Autodesk Fusion 360 part; units mm, degrees
sketch "Sketch1" plane through (0, 0, 0) normal (0, 1, 0) x (1, 0, 0)
  line L0 (0, 0) -> (50, 0)
  line L1 (50, 0) -> (50, -50)
  line L2 (50, -50) -> (0, -50)
  line L3 (0, -50) -> (0, 0)
  dimension "d1" = 50
  dimension "d2" = 50
extrude "Extrude1" add sketch "Sketch1" along normal blind 15
sketch "Sketch2" plane through (0, 15, 0) normal (0, 1, 0) x (-1, 0, 0)
  line L0 (0, 50) -> (-50, 50)
  line L1 (-50, 50) -> (-50, 0)
  line L2 (-50, 0) -> (0, 0)
  line L3 (0, 0) -> (0, 50)
  line L4 (-25, 50) -> (-25, 0) construction
  line L5 (0, 25) -> (-50, 25) construction
  line L6 (-46.6959, 41.7465) -> (-42.6959, 41.7465)
  line L7 (-42.6959, 41.7465) -> (-42.6959, 46.7465)
  line L8 (-42.6959, 46.7465) -> (-46.6959, 46.7465)
  line L9 (-46.6959, 46.7465) -> (-46.6959, 41.7465)
  line L10 (-42.6959, 3.2535) -> (-46.6959, 3.2535)
  line L11 (-46.6959, 3.2535) -> (-46.6959, 8.2535)
  line L12 (-46.6959, 8.2535) -> (-42.6959, 8.2535)
  line L13 (-42.6959, 8.2535) -> (-42.6959, 3.2535)
  line L14 (-3.3041, 41.7465) -> (-7.3041, 41.7465)
  line L15 (-3.3041, 46.7465) -> (-3.3041, 41.7465)
  line L16 (-7.3041, 41.7465) -> (-7.3041, 46.7465)
  line L17 (-7.3041, 46.7465) -> (-3.3041, 46.7465)
  line L18 (-7.3041, 8.2535) -> (-7.3041, 3.2535)
  line L19 (-3.3041, 8.2535) -> (-7.3041, 8.2535)
  line L20 (-3.3041, 3.2535) -> (-3.3041, 8.2535)
  line L21 (-7.3041, 3.2535) -> (-3.3041, 3.2535)
  dimension "d5" = 5
  dimension "d6" = 4
extrude "Extrude2" add sketch "Sketch2" along normal blind 50 contours L6 L7 L8 L9 | L10 L11 L12 L13 | L14 L15 L16 L17 | L18 L19 L20 L21
fillet "Fillet1" radius 5 1 edges at (0, 0, 25)
sketch "Sketch3" plane through (0, 0, 0) normal (0, -1, 0) x (1, 0, 0)
  line L0 (5, 50) -> (5, 0)
  line L1 (5, 0) -> (50, 0)
  line L2 (50, 0) -> (50, 50)
  line L3 (50, 50) -> (5, 50)
  line L4 (50, 0) -> (45, 0)
  line L5 (45, 0) -> (45, 50)
  line L6 (45, 50) -> (50, 50)
  line L7 (50, 50) -> (50, 0)
  dimension "d11" = 5
  dimension "d12" = 50
extrude "Extrude3" add sketch "Sketch3" along normal blind 50 contours L1 L2 L3 L4 L5 L6 L7
The listing builds one solid part. Answer for the finished solid, in the listing's coordinates (mm). A direction names the side the tool comes from. Coordinates: 2 decimals unless noted, no trailing zeros. Write each loop counter-clockwise with the first axis right and the second up, starting at its lowest first coordinate (ties: lowest second). Pieces come first, ordered by that corner, then holes. Notation, with made-up numbers: M 85,-12 L 142,-12 A12 cw 142,0 Z; hole C 79.25,16.25 d11. An arc over 180 degrees is marked long. Put each result on its own line as item: value. Start each with the question number.
1. Consider line 1 (Z direction, x = 4.5, y = 33.5); line 2 (Y direction, x = 11.5, z = 31); line 3 (X direction, y = -12, z = 9). Determine where each line is inside the solid, lowest interval first. Write a range as from..to.
2. A cutting plane is placed at A-A on y = 19. Write down the section's boundary in (x, z).
3. A cutting plane is placed at D-D on x = 23.5. Write down the section's boundary in (y, z).
4. Flat-ended cylindrical pins translate along their axes: P1, Ø2.5, axis at y = 30.5, z = 44.5, coming from the +X side; P2, Ø1.5, axis at y = 39.5, z = 5, coming from the -X side; P3, Ø2, axis at x = 5, y = 29.5, coming from the -Z side; P4, Ø12, axis at y = 26.5, z = 34.5, coming from the +X side. Find the tip coordinate at first contact, or state that the pin passes through.
5. A cutting plane is placed at B-B on z = 29.5. Write down the section's boundary in (x, y).
6. For a pull along X with two mould halves and no side action, classify faces 4 (the flat face through (7.304, 40, 44)), 5 (the flat face through (46.696, 40, 44)), 6 (the flat face through (45, 40, 46.746)), 7 (the flat face through (45, -25, 25)) as pulls with the +X half, pulls with the -X half, needs draft (parallel to the pull), parting line crosses it, or undercut.
7. Which of the six approach directions +Z, -Z, +X, -X, +Y, -Y give full straight-line access (tool end or side, diameter ignored) to faces 1 (the flat face through (3.304, 40, 44)), 2 (the flat face through (46.696, 40, 6)), 3 (the flat face through (5, 40, 41.746))?
8. A cutting plane is placed at C-C on y = -11.5. Write down the section's boundary in (x, z), then the cut area to 3 significant figures.
Resolved:
1. line 1: z = 3.25..8.25, 41.75..46.75
1. line 2: y = 0..15
1. line 3: x = 45..50
2. outline: M 3.3,3.25 L 7.3,3.25 L 7.3,8.25 L 3.3,8.25 Z; M 3.3,41.75 L 7.3,41.75 L 7.3,46.75 L 3.3,46.75 Z; M 42.7,3.25 L 46.7,3.25 L 46.7,8.25 L 42.7,8.25 Z; M 42.7,41.75 L 46.7,41.75 L 46.7,46.75 L 42.7,46.75 Z
3. outline: M 0,0 L 15,0 L 15,50 L 0,50 Z
4. P1: stops at x = 46.7
4. P2: stops at x = 3.3
4. P3: stops at z = 3.25
4. P4: passes through
5. outline: M 0,5 A5 ccw 5,0 L 45,0 L 45,-50 L 50,-50 L 50,15 L 0,15 Z
6. face 4: undercut
6. face 5: pulls with the +X half
6. face 6: needs draft
6. face 7: pulls with the -X half
7. face 1: +Z, -Z, -X, +Y
7. face 2: +Z, -Z, +X, +Y
7. face 3: +X, -X, +Y
8. outline: M 45,0 L 50,0 L 50,50 L 45,50 Z
8. area: 250 mm2
